Input: part model. Units: mm. Frame: model coordinates. A direction names the side the tool comes from. Coordinates: 2 decimals unless noted, no trailing zeros. Loops run counter-clockwise (first coordinate to the right, second up) from the corner with the lowest first, then second, coordinate; pieces in that order, holes last.
Item 1: Contact query for flat-ended pins moving along their axis: P1, Ø4, axis at x = -10.5, y = 11, coming from the -Z side; P2, Ø5, axis at y = 4, z = 40, coming from the +X side; P3, Ø3, axis at x = -12, z = 20.5, coming from the +Y side. Output: stop coordinate, or through.
Item 2: Ray query, line 1 along X through (y, z) = (7.75, 0); line 2 along Z through (x, y) = (-0.5, 5.5); line 3 along X through (y, z) = (3.75, 5.5). Return the intervals inside material, ascending.
Item 3: Section B-B on x = 0. Return loops of the section in (y, z).
Item 4: Reachability of faces 1 (the cylindrical face through (3.755, 7.395, 11.923)), 2 (the cylindrical face through (14.19, 7.9, -20.71)) from +Z, -Z, +X, -X, +Y, -Y: full face, straight path, thin tool, end or side. Return the list, or none.
Item 5: Section C-C on y = 8.5. Return loops of the section in (x, z).
Item 6: Section A-A on z = 0. Return loops of the section in (x, y).
Item 7: Section D-D on x = -42. Return loops of the section in (y, z), and give its area (3 significant figures).
Item 8: Pull-direction query (X, two-part tool) for faces 3 (the cylindrical face through (15.77, 7.395, 50.076)), 4 (the flat face through (-11, 0, 11)), 5 (the cylindrical face through (-25.714, 8.096, -0.622)); classes: released by +X, released by -X, zero draft, split by the parting line, or undercut.
```python
from build123d import *

# Parameters (mm, degrees)
SKETCH1_R             = 52.5
BOSS_EXTRUDE1_DEPTH   = 15
SKETCH2_R             = 12.5
CUT_EXTRUDE1_DEPTH    = 76.746287038
SKETCH3_R             = 2.868901353
CUT_EXTRUDE2_DEPTH    = 14.003451
CIRPATTERN1_START     = 0.996548717
CIRPATTERN1_OUTLINE_R = 2.868901353
CIRPATTERN1_DEPTH     = 14.003451283


# Read off the part's stored shape, not the designer's step: CirPattern1
with BuildPart() as part:
    # Sketch1 → Boss-Extrude1 (new body)
    with BuildSketch(Plane(origin=(0, 0, 0), x_dir=(1, 0, 0), z_dir=(0, 1, 0))):
        with Locations(Location((0, 0, 0), (0, 0, 270))):
            Circle(SKETCH1_R)
    extrude(amount=BOSS_EXTRUDE1_DEPTH)

    # Sketch2 → Cut-Extrude1 (cut, through all)
    with BuildSketch(Plane(origin=(0, 0, 0), x_dir=(1, 0, 0), z_dir=(0, 1, 0))):
        with Locations(Location((0, 0, 0), (0, 0, 270))):
            Circle(SKETCH2_R)
    extrude(amount=CUT_EXTRUDE1_DEPTH, mode=Mode.SUBTRACT)

    # Sketch3 → Cut-Extrude2 (cut)
    with BuildSketch(Plane(origin=(0, 15, 0), x_dir=(1, 0, 0), z_dir=(0, 1, 0))):
        with Locations(Location((-22.913471565, 0, 0), (0, 0, 270))):
            Circle(SKETCH3_R)
    extrude(amount=-CUT_EXTRUDE2_DEPTH, mode=Mode.SUBTRACT)

    # CirPattern1 outline → CirPattern1 (cut)
    with BuildSketch(Plane(origin=(0, 0, 0), x_dir=(1, 0, 0), z_dir=(0, 1, 0)).offset(CIRPATTERN1_START)):
        with Locations((-11.456735782, -19.843648464)):
            Circle(CIRPATTERN1_OUTLINE_R)
        with Locations((11.456735782, -19.843648464)):
            Circle(CIRPATTERN1_OUTLINE_R)
        with Locations((22.913471565, 0)):
            Circle(CIRPATTERN1_OUTLINE_R)
        with Locations((11.456735782, 19.843648464)):
            Circle(CIRPATTERN1_OUTLINE_R)
        with Locations((-11.456735782, 19.843648464)):
            Circle(CIRPATTERN1_OUTLINE_R)
    extrude(amount=CIRPATTERN1_DEPTH, mode=Mode.SUBTRACT)


solid = part.part
```
Results found:
1. P1: stops at z = -51.81
1. P2: stops at x = 36.74
1. P3: stops at y = 1
2. line 1: x = -52.5 to -25.78, -20.04 to -12.5, 12.5 to 20.04, 25.78 to 52.5
2. line 2: z = -52.5 to -12.49, 12.49 to 52.5
2. line 3: x = -52.21 to -11.22, 11.22 to 52.21
3. outline: (0, -52.5) - (15, -52.5) - (15, -12.5) - (0, -12.5) - close; (0, 12.5) - (15, 12.5) - (15, 52.5) - (0, 52.5) - close
4. face 1: +Y, -Y
4. face 2: +Y
5. outline: circle Ø105 at (0, 0); hole circle Ø5.74 at (-22.91, 0); hole circle Ø5.74 at (-11.46, -19.84); hole circle Ø5.74 at (-11.46, 19.84); hole circle Ø25 at (0, 0); hole circle Ø5.74 at (11.46, -19.84); hole circle Ø5.74 at (11.46, 19.84); hole circle Ø5.74 at (22.91, 0)
6. outline: (-52.5, 0) - (-12.5, 0) - (-12.5, 15) - (-20.04, 15) - (-20.04, 1) - (-25.78, 1) - (-25.78, 15) - (-52.5, 15) - close; (12.5, 0) - (52.5, 0) - (52.5, 15) - (25.78, 15) - (25.78, 1) - (20.04, 1) - (20.04, 15) - (12.5, 15) - close
7. outline: (0, -31.5) - (15, -31.5) - (15, 31.5) - (0, 31.5) - close
7. area: 945 mm2
8. face 3: split by the parting line
8. face 4: zero draft
8. face 5: undercut
